Autodesk Inventor part; units mm, degrees
sketch "Base" plane through (0, 0, 0) normal (0, 1, 0) x (-1, 0, 0)
  arc A0 (16.4327, -16.6683) -> (16.4327, -3.9692) centre (16.3612, -10.3188) ccw
  circle A1 centre (16.3612, -10.3188) radius 6.35
  point P0 (0, 0)
extrude "ForwardFeature" add sketch "Base" along normal blind 309.88 draft -0.5
sketch "Sketch2" plane through (-16.3612, 0, -10.3188) normal (0, -1, 0) x (1, 0, 0)
  circle A0 centre (0, 0) radius 6.35
  point P0 (16.3612, 10.3188)
extrude "BackFeature" add sketch "Sketch2" along normal blind 88.9
sketch "Sketch3" plane through (0, 0, 0) normal (0, 1, 0) x (-1, 0, 0)
  arc A0 (16.2898, 3.9686) -> (16.4327, 3.9686) centre (16.3612, -10.3188) ccw construction
  circle A1 centre (16.3612, -10.3188) radius 14.2875
  point P0 (0, 0)
extrude "CollarFeature" add sketch "Sketch3" along normal mid plane 10.16
properties part number "DrumstickBoundingBox"
Design review of the part built by this model. Coordinates are the model's own, in mm. A direction names the side the tool comes from. Give positions to 0.01 mm unless a question says otherwise; leave off trailing zeros. Order: outer loops, then holes, each group sorted by start corner. A loop starts at its lowest first (then second) coordinate and runs counter-clockwise, first axis right, second up. Notation, with made-up numbers: M 49.25,-1 L 75.25,-1 A29 cw 75.25,25 Z; hole C 61,-15 d11. An arc over 180 degrees is marked long. One line per question, with ' | ' between items. Start each with the question number.
Q1. We need section A-A (z = 0). Write out the cut boundary in (x, y).
Q2. We need section B-B (y = 16). Write out the cut boundary in (x, z).
Q3. We need section D-D (y = 246). Write out the cut boundary in (x, z), plus the area to 3 significant figures.
Q4. For L1, parallel to Y at x = -19.25, z = -18.5; L2, parallel to X at y = -61.5, z = -12.5; L3, parallel to X at y = 119.5, z = -11.5, list the stretches that pass through material, from the lowest coordinate up. Write a range as [from, to].
Q5. For pin 1 Ø4 at (y, z) = (162.5, -9.5) entering from -X; pin 2 Ø3 at (y, z) = (213, -12) entering from +X; pin 3 Ø1.5 at (x, z) = (-5, -16) entering from -Y, all flat-tipped, find the tip position at first contact; note any pin that passes through.
Q6. We need section C-C (x = -26.5). Write out the cut boundary in (y, z).
Q7. Machinability: for faces 1 (the face through (-23, 5.08, -13)), 2 (the face through (-16, 309.88, -10)), 3 (the face through (-23, -5.08, -13)), which of the approach directions +Z, -Z, +X, -X, +Y, -Y give a long, thin tool a straight path to every point of the face, cutting with its end or side? Answer none if there is none.
Returned:
1) outline: M -26.24,-5.08 L -6.48,-5.08 L -6.48,5.08 L -26.24,5.08 Z
2) outline: M -16.43,-16.53 A6.21 ccw long -16.43,-4.11 A6.21 ccw Z
3) outline: M -16.41,-14.52 A4.2 ccw long -16.41,-6.12 A4.2 ccw Z | area: 55.5 mm2
4) L1: [-5.08, 5.08] | L2: [-22.32, -10.4] | L3: [-21.54, -11.19]
5) pin 1: x = -21.31 | pin 2: x = -11.87 | pin 3: y = -5.08
6) outline: M -5.08,-20.39 L 5.08,-20.39 L 5.08,-0.25 L -5.08,-0.25 Z
7) face 1: +Y | face 2: +Z, -Z, +X, -X, +Y | face 3: -Y
